Can you work these out from the model? Positions are in its coordinate system, mm. A direction names the side the tool comes from. Give positions to 0.01 mm unless a question says otherwise; leave off trailing zeros. Order: outer loops, then holes, each group sorted by start corner. A loop starts at its lowest first (then second) coordinate and runs counter-clockwise, first axis right, second up. Notation, with made-up numbers: (88, 88.5) - (117, 88.5) arc R34 ccw to (117, 123.5) - close; hole circle Ø8 at (38, 42.5). An arc over 180 degrees is marked (long way). Use one line per item in the form item = value. Start each with the question number.
1) Which directions (+Z, -Z, +X, -X, +Y, -Y) give clear straight access to the entire face, cutting with the end or side of a thin tool? Please do faces 1 (the flat face through (12.5, 0.2, 0.1)), 2 (the flat face through (-3.181, -0.5, 0)), 3 (the flat face through (0, 1.5, -5)), 4 (the flat face through (0, -1, 0)).
2) Please list where these lines run through material, in increasing order: probe 1 along X at (y, z) = (-0.5, 4.25); probe 2 along Z at (x, y) = (20.5, 1); probe 3 along Y at (x, z) = (-0.5, 3.75).
3) For pin 1 (5 mm diameter, centred on x = -16.5, z = -1.5, fed in from +Y); pin 2 (4 mm diameter, centred on x = 1, z = -3, fed in from -Y); pin 3 (6 mm diameter, centred on x = -17.5, z = -2.5, fed in from -Y); pin 4 (4 mm diameter, centred on y = -1.5, z = 0.5, fed in from +X), each with a flat end and sliding along its axis, tell me the tip position at first contact or that it passes through.
4) Suppose I cut it at B-B, the plane y = -2. Write out the boundary of the cut face in (x, z), and give its area (3 significant figures).
5) We'd pull the mould along Z, two halves only. Please class faces 5 (the cylindrical face through (-7.715, 1.993, 3.699)), 6 (the cylindrical face through (-17.43, 2.095, 1.422)), 7 (the flat face through (0, 2.5, 0)), 8 (the flat face through (-12.5, 2.23, -4.24)): released by +Z, released by -Z, zero draft, split by the parting line, or undercut.
```python
from build123d import *

# Parameters (mm, degrees)
SKETCH1_W            = 25
SKETCH1_H            = 12
BOSS_EXTRUDE1_DEPTH  = 1.5
SKETCH2_R            = 1
BOSS_EXTRUDE2_DEPTH  = 10
SKETCH3_R            = 0.6
BOSS_EXTRUDE3_DEPTH  = 3
SKETCH4_R            = 1
SKETCH4_R_2          = 0.6
BOSS_EXTRUDE4_DEPTH  = 10
SKETCH5_R            = 0.6
SKETCH5_R_2          = 0.4
BOSS_EXTRUDE5_DEPTH  = 2
BOSS_EXTRUDE6_DEPTH  = 1
SKETCH8_R            = 2.5
BOSS_EXTRUDE10_DEPTH = 11
SKETCH9_W            = 6.362334076
SKETCH9_H            = 5.27029166
BOSS_EXTRUDE11_DEPTH = 1
SKETCH10_W           = 1.899204201
SKETCH10_H           = 1.329442941
SKETCH10_W_2         = 1.614323571
SKETCH10_H_2         = 2.374005252
SKETCH10_W_3         = 3.418567563
SKETCH10_H_3         = 0.85464189
SKETCH10_W_4         = 1.139522521
SKETCH10_W_5         = 1.234482731
SKETCH10_H_4         = 1.804243992
SKETCH10_W_6         = 1.351356835
SKETCH10_W_7         = 3.250561037
SKETCH10_H_5         = 1.187002626
BOSS_EXTRUDE12_DEPTH = 0.8


with BuildPart() as part:
    # Sketch1 → Boss-Extrude1 (new body)
    with BuildSketch(Plane(origin=(0, 0, 0), x_dir=(1, 0, 0), z_dir=(0, 1, 0))):
        Rectangle(SKETCH1_W, SKETCH1_H)
    extrude(amount=BOSS_EXTRUDE1_DEPTH)

    # Sketch2 → Boss-Extrude2 (add)
    with BuildSketch(Plane(origin=(12.5, 0, 0), x_dir=(0, 0, -1), z_dir=(1, 0, 0))):
        with Locations((0, 1.5)):
            Circle(SKETCH2_R)
        with Locations((-4, 1.5)):
            Circle(SKETCH2_R)
        with Locations((4, 1.5)):
            Circle(SKETCH2_R)
    extrude(amount=BOSS_EXTRUDE2_DEPTH)

    # Sketch3 → Boss-Extrude3 (add)
    with BuildSketch(Plane(origin=(12.5, 0, 0), x_dir=(0, 0, -1), z_dir=(1, 0, 0))):
        with Locations((-4, 1.5)):
            Circle(SKETCH3_R)
        with Locations((0, 1.5)):
            Circle(SKETCH3_R)
        with Locations((4, 1.5)):
            Circle(SKETCH3_R)
    extrude(amount=-BOSS_EXTRUDE3_DEPTH)

    # Sketch4 → Boss-Extrude4 (add)
    with BuildSketch(Plane.ZY.offset(12.5)):
        with Locations((-4, 1.5)):
            Circle(SKETCH4_R)
        with Locations((4, 1.5)):
            Circle(SKETCH4_R)
        with Locations((0, 1.5)):
            Circle(SKETCH4_R_2)
        with Locations((1.5, 1.5)):
            Circle(SKETCH4_R_2)
        with Locations((-1.5, 1.5)):
            Circle(SKETCH4_R_2)
    extrude(amount=BOSS_EXTRUDE4_DEPTH)

    # Sketch5 → Boss-Extrude5 (add)
    with BuildSketch(Plane(origin=(-12.5, 0, 0), x_dir=(0, 0, -1), z_dir=(1, 0, 0))):
        with Locations((-4, 1.5)):
            Circle(SKETCH5_R)
        with Locations((-1.5, 1.5)):
            Circle(SKETCH5_R_2)
        with Locations((0, 1.5)):
            Circle(SKETCH5_R_2)
        with Locations((1.5, 1.5)):
            Circle(SKETCH5_R_2)
        with Locations((4, 1.5)):
            Circle(SKETCH5_R)
    extrude(amount=BOSS_EXTRUDE5_DEPTH)

    # Sketch6 → Boss-Extrude6 (add)
    with BuildSketch(Plane(origin=(0, 1.5, 0), x_dir=(1, 0, 0), z_dir=(0, 1, 0))):
        with BuildLine():
            Line((-7, -4), (7, -4))
            ThreePointArc((7, -4), (7.707106781, -3.707106781), (8, -3))
            Line((8, -3), (8, 3))
            ThreePointArc((8, 3), (7.707106781, 3.707106781), (7, 4))
            Line((7, 4), (-7, 4))
            ThreePointArc((-7, 4), (-7.707106781, 3.707106781), (-8, 3))
            Line((-8, 3), (-8, -3))
            ThreePointArc((-8, -3), (-7.707106781, -3.707106781), (-7, -4))
        make_face()
    extrude(amount=BOSS_EXTRUDE6_DEPTH)

    # Sketch8 → Boss-Extrude10 (add)
    with BuildSketch(Plane.XY.offset(5.5)):
        with Locations((-13, -2.05)):
            Circle(SKETCH8_R)
    extrude(amount=-BOSS_EXTRUDE10_DEPTH)

    # Sketch9 → Boss-Extrude11 (add)
    with BuildSketch(Plane.XZ):
        Rectangle(SKETCH9_W, SKETCH9_H)
    extrude(amount=BOSS_EXTRUDE11_DEPTH)

    # Sketch10 → Boss-Extrude12 (add)
    with BuildSketch(Plane.XZ):
        with Locations((-8.688859223, 3.347347405)):
            Rectangle(SKETCH10_W, SKETCH10_H)
        with Locations((-7.406896386, -1.780503939)):
            Rectangle(SKETCH10_W_2, SKETCH10_H_2)
        with Locations((1.471883257, -3.917108666)):
            Rectangle(SKETCH10_W_3, SKETCH10_H_3)
        with Locations((4.415649769, -1.780503939)):
            Rectangle(SKETCH10_W_4, SKETCH10_H_2)
        with Locations((5.887533026, 4.012068876)):
            Rectangle(SKETCH10_W_5, SKETCH10_H_4)
        with Locations((7.823260385, 4.012068876)):
            Rectangle(SKETCH10_W_6, SKETCH10_H_4)
        with Locations((7.823260385, 0)):
            Rectangle(SKETCH10_W_7, SKETCH10_H_5)
    extrude(amount=BOSS_EXTRUDE12_DEPTH)


solid = part.part
```
Result sheet:
q1.face_1 = +X, -Y
q1.face_2 = +Z, -Z, -Y
q1.face_3 = +Y
q1.face_4 = +Z, -Z, +X, -Y
q2.probe_1 = -14.96 to -11.04, 5.27 to 6.5, 7.15 to 8.5
q2.probe_2 = -4.87 to -3.13, -0.87 to 0.87, 3.13 to 4.87
q2.probe_3 = 0 to 2.5
q3.pin_1 = 2.5
q3.pin_2 = -1
q3.pin_3 = -4.05
q3.pin_4 = 12.5
q4.outline = (-15.5, -5.5) - (-10.5, -5.5) - (-10.5, 5.5) - (-15.5, 5.5) - close
q4.area = 55.0 mm²
q5.face_5 = released by +Z
q5.face_6 = undercut
q5.face_7 = zero draft
q5.face_8 = undercut
